from build123d import *

# Parameters (mm, degrees)
SKETCH1_R           = 15.875
BOSS_EXTRUDE1_DEPTH = 22.225
SKETCH1_3_R         = 10.795
CUT_EXTRUDE1_DEPTH  = 5.08
BOSS_EXTRUDE2_START = 5.08
SKETCH1_4_R         = 5.08
BOSS_EXTRUDE2_DEPTH = 0.889
BOSS_EXTRUDE3_START = 5.08
SKETCH1_5_R         = 3.175
BOSS_EXTRUDE3_DEPTH = 6.35
SKETCH2_R           = 3.27025
CUT_EXTRUDE2_DEPTH  = 12.7
SKETCH3_R           = 1.5875
CUT_EXTRUDE4_DEPTH  = 24.495
SKETCH3_3_R         = 1.5875
BOSS_EXTRUDE4_DEPTH = 22.225


with BuildPart() as part:
    # Sketch1 → Boss-Extrude1 (new body)
    with BuildSketch(Plane.XY):
        Circle(SKETCH1_R)
    extrude(amount=BOSS_EXTRUDE1_DEPTH)

    # Sketch1<3> → Cut-Extrude1 (cut)
    with BuildSketch(Plane.XY):
        Circle(SKETCH1_3_R)
    extrude(amount=CUT_EXTRUDE1_DEPTH, mode=Mode.SUBTRACT)

    # Sketch1<4> → Boss-Extrude2 (add)
    with BuildSketch(Plane.XY.offset(BOSS_EXTRUDE2_START)):
        Circle(SKETCH1_4_R)
    extrude(amount=-BOSS_EXTRUDE2_DEPTH)

    # Sketch1<5> → Boss-Extrude3 (add)
    with BuildSketch(Plane.XY.offset(BOSS_EXTRUDE3_START)):
        Circle(SKETCH1_5_R)
    extrude(amount=-BOSS_EXTRUDE3_DEPTH)

    # Sketch2 → Cut-Extrude2 (cut)
    with BuildSketch(Plane.XY.offset(22.225)):
        Circle(SKETCH2_R)
    extrude(amount=-CUT_EXTRUDE2_DEPTH, mode=Mode.SUBTRACT)

    # Sketch3 → Cut-Extrude4 (cut, through all)
    with BuildSketch(Plane.XY.offset(22.225)):
        with Locations((15.875, 0)):
            Circle(SKETCH3_R)
    extrude(amount=-CUT_EXTRUDE4_DEPTH, mode=Mode.SUBTRACT)

    # Sketch3<3> → Boss-Extrude4 (add)
    with BuildSketch(Plane.XY.offset(22.225)):
        with Locations((-15.875, 0)):
            Circle(SKETCH3_3_R)
    extrude(amount=-BOSS_EXTRUDE4_DEPTH)


solid = part.part
Verification items for the finished model (mm, model axes). A direction names the side the tool comes from. Coordinates: 2 decimals unless noted, no trailing zeros. Write each loop counter-clockwise with the first axis right and the second up, starting at its lowest first coordinate (ties: lowest second). Pieces come first, ordered by that corner, then holes. Notation, with made-up numbers: (47.25, -12.75) -> (52.25, -12.75) arc R32 ccw to (52.25, 19.25) -> close; hole circle Ø1 at (12, 33.25). An arc over 180 degrees is marked (long way). One line per item, written item: value. Start each with the question number.
Q1. Cross-section at C-C on y = 0. Enter the section's corners in (x, z) (1 decimal), and give its area (3 significant figures).
Q2. Thickness scan on L1, parallel to Y at x = 0, z = 12.25 (3 decimals); L2, parallel to Y at x = 0, z = 3.3 (3 decimals); L3, parallel to Z at x = 14, y = 1.5 (3 decimals). Record the ranges inside material, lowest first. Write a range as from..to.
Q3. Go/stop test with flat-tipped pins: P1, Ø3, axis at x = -12, z = 4, coming from the +Y side; P2, Ø2, axis at y = -7, z = 2.5, coming from the +X side; P3, Ø1, axis at x = -13, z = 2.5, coming from the -Y side; P4, Ø4, axis at x = -13.5, y = -12.5, coming from the -Z side. Record where each tip stops, or that it passes through.
Q4. Cross-section at A-A on x = 0. Enter the section's corners in (y, z) (3 decimals).
Q5. Access from +Z, -Z, +X, -X, +Y, -Y to the whole of each face (thin tool, end or side, straight path). Record for faces 5 (the flat face through (3.3, -1.1, 4.191)), 6 (the cylindrical face through (14.288, 0.034, 11.268)), 7 (the cylindrical face through (-0.43, 3.24, 15.96)).
Q6. Mould release check, pull along X, two halves, no side actions. Record for faces 1 (the cylindrical face through (0.33, 15.87, 10.96)), 2 (the flat face through (0, 0, 9.525)), 3 (the flat face through (-1.1, -3.3, 22.225)), 4 (the cylindrical face through (-0.69, -3.1, 1.5)): pulls with the +X half, pulls with the -X half, needs draft (parallel to the pull), parting line crosses it, or undercut.
Checked values:
1. outline: (-17.5, 0) -> (-10.8, 0) -> (-10.8, 5.1) -> (-5.1, 5.1) -> (-5.1, 4.2) -> (-3.2, 4.2) -> (-3.2, -1.3) -> (3.2, -1.3) -> (3.2, 4.2) -> (5.1, 4.2) -> (5.1, 5.1) -> (10.8, 5.1) -> (10.8, 0) -> (14.3, 0) -> (14.3, 22.2) -> (3.3, 22.2) -> (3.3, 9.5) -> (-3.3, 9.5) -> (-3.3, 22.2) -> (-17.5, 22.2) -> close
1. area: 557 mm²
2. L1: y = -15.875..-3.27, 3.27..15.875
2. L2: y = -15.875..-10.795, -3.175..3.175, 10.795..15.875
2. L3: z = 0..22.225
3. P1: stops at y = 11.91
3. P2: stops at x = 14.7
3. P3: stops at y = -9.79
3. P4: passes through
4. outline: (-15.875, 0) -> (-10.795, 0) -> (-10.795, 5.08) -> (-5.08, 5.08) -> (-5.08, 4.191) -> (-3.175, 4.191) -> (-3.175, -1.27) -> (3.175, -1.27) -> (3.175, 4.191) -> (5.08, 4.191) -> (5.08, 5.08) -> (10.795, 5.08) -> (10.795, 0) -> (15.875, 0) -> (15.875, 22.225) -> (3.27, 22.225) -> (3.27, 9.525) -> (-3.27, 9.525) -> (-3.27, 22.225) -> (-15.875, 22.225) -> close
5. face 5: -Z
5. face 6: +Z, -Z, +X
5. face 7: +Z
6. face 1: parting line crosses it
6. face 2: undercut
6. face 3: needs draft
6. face 4: undercut
